Input: dimensioned drawing with shaded views. Units: mm. Origin: part minimum x, y, z. A direction names the side the tool comes from. Give positions to 0.01 mm unless a question says otherwise; leave off trailing zeros. Loops run counter-clockwise (first coordinate to the right, second up) from the corner with the lowest first, then second, coordinate; pieces in that order, holes last.
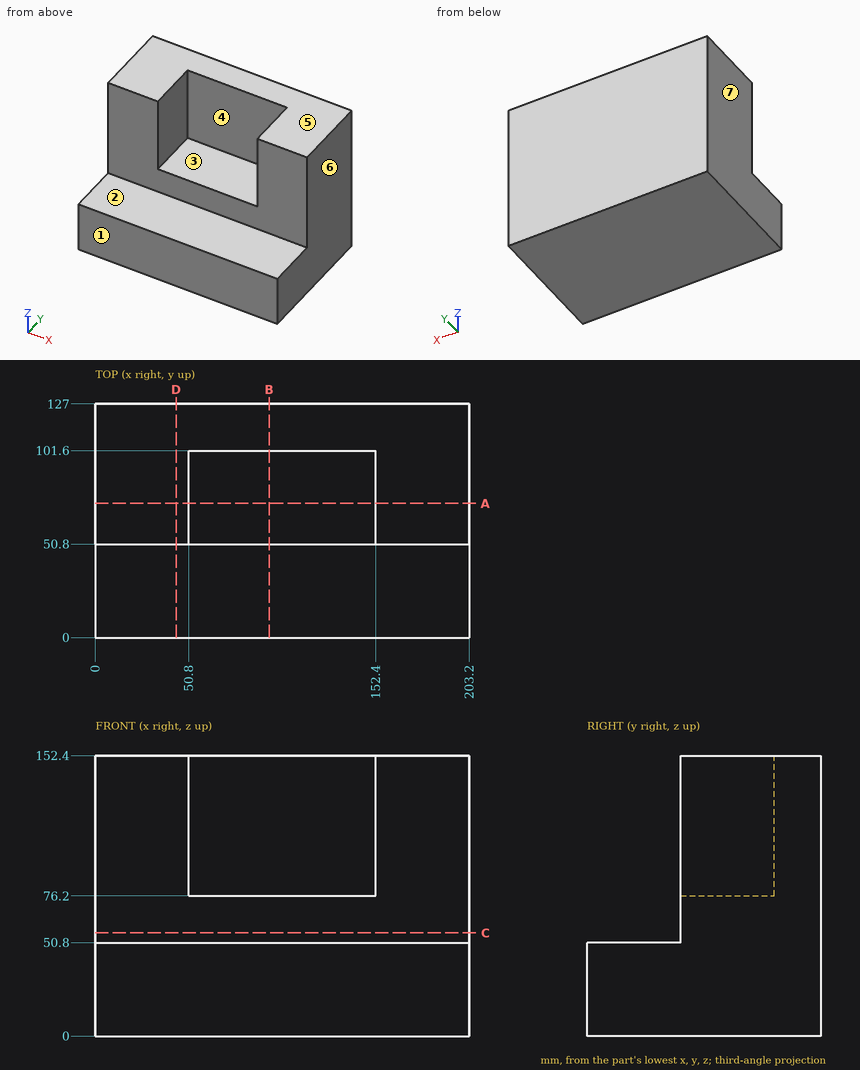
(1) Section A-A, the plane y = 73. Return the cut outline in (x, z).
A:
outline: (0, 0) - (203.2, 0) - (203.2, 152.4) - (152.4, 152.4) - (152.4, 76.2) - (50.8, 76.2) - (50.8, 152.4) - (0, 152.4) - close
(2) Section B-B, the plane x = 94.5. Return the cut outline in (y, z).
A:
outline: (0, 0) - (127, 0) - (127, 152.4) - (101.6, 152.4) - (101.6, 76.2) - (50.8, 76.2) - (50.8, 50.8) - (0, 50.8) - close
(3) First-contact query: pin 1 (3 mm diameter, centred on x = 112.5, y = 33.5, fed in from +Z); pin 2 (8 mm diameter, centred on x = 178.5, z = 109, fed in from -Y). Flat tips, straight axial feed; report the tip coordinate or a pass-through.
A:
pin 1: stops at z = 50.8
pin 2: stops at y = 50.8
(4) Section C-C, the plane z = 56. Return the cut outline in (x, y).
A:
outline: (0, 50.8) - (203.2, 50.8) - (203.2, 127) - (0, 127) - close
(5) Ray query, line 1 along X through (y, z) = (67.5, 116); line 2 along Z through (x, y) = (112, 41); line 3 along Y through (x, z) = (110.5, 129). Return the intervals inside material, ascending.
A:
line 1: x = 0 to 50.8, 152.4 to 203.2
line 2: z = 0 to 50.8
line 3: y = 101.6 to 127
(6) Mould query, pull axis X, two halves, no side actions, for the marked faces 4, 5, 6 and 7. Classes: pulls with the +X half, pulls with the -X half, needs draft (parallel to the pull), parting line crosses it, or undercut.
A:
face 4: undercut
face 5: needs draft
face 6: pulls with the +X half
face 7: pulls with the -X half
(7) Reachability of the marked faces 1, 2 and 3 from +Z, -Z, +X, -X, +Y, -Y: full face, straight path, thin tool, end or side. Return the list, or none.
A:
face 1: +Z, -Z, +X, -X, -Y
face 2: +Z, +X, -X, -Y
face 3: +Z, -Y
(8) Section D-D, the plane x = 44. Return the cut outline in (y, z).
A:
outline: (0, 0) - (127, 0) - (127, 152.4) - (50.8, 152.4) - (50.8, 50.8) - (0, 50.8) - close
